from build123d import *

# Parameters (mm, degrees)
F1_DEPTH = 7.62
F2_R     = 3.80999
F3_R     = 3.80999
F4_R     = 1.27
F5_R     = 1.27


# Not quite as in the source:
# - a fillet or chamfer is up to 0.001 mm smaller than in the source, because OpenCascade refuses the exact size


with BuildPart() as f1:
    # F0 (on Front) → F1 (new body)
    with BuildSketch(Plane.XZ):
        with BuildLine():
            Line((134.7724028379, 37.2032584392), (-111.6075971621, 37.2032584392))
            Line((-111.6075971621, 37.2032584392), (-111.6075971621, 41.0132584392))
            ThreePointArc((-111.6075971621, 41.0132584392), (-110.4916739984, 43.7073352756), (-107.7975971621, 44.8232584392))
            Line((-107.7975971621, 44.8232584392), (-73.5075971621, 44.8232584392))
            Line((-73.5075971621, 44.8232584392), (-73.5075971621, 52.4432584392))
            Line((-73.5075971621, 52.4432584392), (-107.7975971621, 52.4432584392))
            ThreePointArc((-107.7975971621, 52.4432584392), (-115.8798276711, 49.0954889482), (-119.2275971621, 41.0132584392))
            Line((-119.2275971621, 41.0132584392), (-119.2275971621, 37.2032584392))
            Line((-119.2275971621, 37.2032584392), (-119.2275971621, 34.0282584392))
            Line((-119.2275971621, 34.0282584392), (134.7724028379, 34.0282584392))
            Line((134.7724028379, 34.0282584392), (134.7724028379, 37.2032584392))
        make_face()
    extrude(amount=F1_DEPTH)

    # F2 (radius 3.81 in the source; OpenCascade refuses exactly that, so slightly less here)
    f2_edges = [f1.edges().sort_by_distance(p)[0] for p in [
        (-90.652597, -7.62, 52.443258),
        (-90.652597, -7.62, 44.823258),
        (-90.652597, 0, 44.823258),
        (-90.652597, 0, 52.443258),
    ]]
    fillet(f2_edges, radius=F2_R)

    # F3 (radius 3.81 in the source; OpenCascade refuses exactly that, so slightly less here)
    f3_edges = [f1.edges().sort_by_distance(p)[0] for p in [
        (-73.507597, -3.81, 52.443258),
        (-73.507597, -1.11592, 51.327338),
        (-73.507597, 0, 48.633258),
        (-73.507597, -1.11592, 45.939179),
        (-73.507597, -3.81, 44.823258),
        (-73.507597, -6.50408, 45.939179),
        (-73.507597, -6.50408, 51.327338),
        (-73.507597, -7.62, 48.633258),
    ]]
    fillet(f3_edges, radius=F3_R)

    # F4
    f4_edges = [f1.edges().sort_by_distance(p)[0] for p in [
        (11.582403, -7.62, 37.203258),
        (9.677398, -7.62, 34.028258),
        (11.582403, 0, 37.203258),
        (9.677398, 0, 34.028258),
    ]]
    fillet(f4_edges, radius=F4_R)

    # F5
    f5_edges = [f1.edges().sort_by_distance(p)[0] for p in [
        (134.772403, -7.248026, 36.831284),
        (134.772403, -7.62, 35.615758),
        (134.772403, -7.248026, 34.400233),
        (134.772403, -3.81, 34.028258),
        (134.772403, -0.371974, 34.400233),
        (134.772403, 0, 35.615758),
        (134.772403, -3.81, 37.203258),
        (134.772403, -0.371974, 36.831284),
    ]]
    fillet(f5_edges, radius=F5_R)


solid = f1.part
Geometry check sheet. Reference: the model listing, model coordinates, mm. Round coordinates to 2 decimals unless told otherwise and drop trailing zeros. Loops run counter-clockwise (first coordinate to the right, second up) from the corner with the lowest first, then second, coordinate; pieces in that order, holes last. Notation, with made-up numbers: (83.25, 21.25) -> (87.25, 21.25) arc R13 ccw to (87.25, 27.25) -> close; hole circle Ø5 at (-37, -1.75). An arc over 180 degrees is marked (long way). Answer as a JSON object with one key per item and string values. Group by question number.
Item 1: Thickness scan on line 1 along Z through (x, y) = (0, -4); line 2 along Z through (x, y) = (-105.5, -5.5); line 3 along Z through (x, y) = (-89, -5.25). Record the ranges inside material, lowest first.
Item 2: Cross-section at A-A, the plane x = -39. Record the cut outline in (y, z).
Item 3: Depth check by flat-ended pin: pin 1 Ø1.5 at (x, y) = (5.5, -5) entering from +Z; pin 2 Ø10 at (x, z) = (-74, 42.5) entering from -Y. Enter the tip coordinate at first touch or a pass-through.
Determined:
{
 "1": {"line 1": "z = 34.03 to 37.2", "line 2": "z = 34.03 to 37.2, 45.22 to 52.05", "line 3": "z = 34.03 to 37.2, 45.11 to 52.16"},
 "2": {"outline": "(-7.62, 35.3) arc R1.27 ccw to (-6.35, 34.03) -> (-1.27, 34.03) arc R1.27 ccw to (0, 35.3) -> (0, 35.93) arc R1.27 ccw to (-1.27, 37.2) -> (-6.35, 37.2) arc R1.27 ccw to (-7.62, 35.93) -> close"},
 "3": {"pin 1": "stops at z = 37.2", "pin 2": "stops at y = -7.07"}
}
